The listing builds one solid part. Answer for the finished solid, in the listing's coordinates (mm). Give positions to 0.01 mm unless a question says otherwise; leave off trailing zeros. Loops run counter-clockwise (first coordinate to the right, second up) from the corner with the lowest first, then second, coordinate; pieces in that order, holes last. Notation, with made-up numbers: (68, 35.5) - (106, 35.5) arc R18 ccw to (106, 62.5) - close; hole circle Ø8 at (71, -37.5). An arc over 180 degrees is marked (long way). Write item = value, one per line. Start each with the question number.
1) The part is cut by section A-A on x = 0. Write down the section's boundary in (y, z), plus the area to 3 significant figures.
2) The part is cut by section D-D on z = 0.8. State how many separate pieces and enclosed holes the cut face has, plus the area to 3 significant figures.
3) The part is cut by section C-C on x = -22.5. Write down the section's boundary in (y, z).
4) Consider probe 1 along Y at (x, z) = (-30, 0.95); probe 2 along X at (y, z) = (31, 0.9); probe 3 along Y at (x, z) = (-39.5, 0.1). Determine where each line is inside the solid, lowest interval first.
5) The mould has two halves that part along Y. Classify faces 1 (the flat face through (33, -19, 0)), 2 (the cylindrical face through (-21.77, 32.96, 0.51)): +Y half, -Y half, draft (parallel to the pull), parting line (faces both ways), or undercut.
from build123d import *

# Parameters (mm, degrees)
SKETCH_R           = 44.3
SKETCH_R_2         = 38
PAD_DEPTH          = 1
POCKET_DEPTH       = 251.607624
POLARPATTERN_COUNT = 16


with BuildPart() as part:
    # Sketch → Pad (new body)
    with BuildSketch(Plane.XY):
        Circle(SKETCH_R)
        with Locations((-0.109724, 0)):
            Circle(SKETCH_R_2, mode=Mode.SUBTRACT)
    extrude(amount=PAD_DEPTH)

    # Sketch001 → Pocket (cut, through all)
    with BuildSketch(Plane.XY.offset(1)):
        with BuildLine():
            ThreePointArc((42.878892, -3.225), (43, 0), (42.878892, 3.225))
            Line((0, 0), (42.878892, 3.225))
            Line((0, 0), (42.878892, -3.225))
        make_face()
        with BuildLine():
            ThreePointArc((41.730018, 4.754535), (41.228342, 8.013978), (40.472479, 11.224012))
            Line((40.472479, 11.224012), (38.063403, 10.555916))
            ThreePointArc((39.246088, 4.471527), (38.774274, 7.536955), (38.063403, 10.555916))
            Line((41.730018, 4.754535), (39.246088, 4.471527))
        make_face()
    pocket = extrude(amount=-POCKET_DEPTH, mode=Mode.SUBTRACT)

    # PolarPattern: Pocket ×16 about axis
    polarpattern_axis = Axis((0, 0, 1), (0, 0, 1))
    for i in range(1, POLARPATTERN_COUNT):
        add(pocket.rotate(polarpattern_axis, i * 360 / POLARPATTERN_COUNT), mode=Mode.SUBTRACT)


solid = part.part
Answer below:
q1.outline = (-44.3, 0) - (-43, 0) - (-43, 1) - (-44.3, 1) - close; (43, 0) - (44.3, 0) - (44.3, 1) - (43, 1) - close
q1.area = 2.60 mm2
q2.separate_pieces = 1
q2.enclosed_holes = 17
q2.area = 886 mm2
q3.outline = (-38.16, 0) - (-35.46, 0) - (-35.46, 1) - (-38.16, 1) - close; (-32.47, 0) - (-30.7, 0) - (-30.7, 1) - (-32.47, 1) - close; (30.7, 0) - (32.47, 0) - (32.47, 1) - (30.7, 1) - close; (35.46, 0) - (38.16, 0) - (38.16, 1) - (35.46, 1) - close
q4.probe_1 = -32.6 to -30.81, -25.8 to -23.46, 23.46 to 25.8, 30.81 to 32.6
q4.probe_2 = -31.65 to -29.8, -26.66 to -22.09, 21.87 to 24.48, 24.66 to 26.66, 29.8 to 31.65
q4.probe_3 = -20.06 to -16.99, -12.99 to -10.95, -4.5 to -2.97, 2.97 to 4.85, 11.33 to 12.99, 16.99 to 20.06
q5.face_1 = draft
q5.face_2 = undercut
